Read the model definition and answer for the solid it produces. Units are mm, in the model's axes. A direction names the side the tool comes from. Give positions to 0.01 mm unless a question says otherwise; leave off trailing zeros. Loops run counter-clockwise (first coordinate to the right, second up) from the corner with the lowest first, then second, coordinate; pieces in that order, holes last. Notation, with made-up numbers: (-3, 31.25) - (37, 31.25) arc R3 cw to (37, 35.25) - close; hole circle Ø1 at (25.5, 43). An arc over 180 degrees is marked (long way). Put each result on its own line as item: value. Start each with the question number.
1. A cutting plane is placed at D-D, the plane y = -11. Determine the outline of the cut face in (x, z) (3 decimals), plus the area to 3 significant figures.
2. Given pin 1 Ø1 at (x, z) = (-6, 3) entering from -Y; pin 2 Ø3 at (y, z) = (-10.5, 7) entering from -X; pin 3 Ø1.5 at (y, z) = (4, 5.5) entering from +X; pin 4 Ø3.5 at (x, z) = (-1.5, 7) entering from +Y (3 decimals), each flat-ended and moving along its own axis, determine where each tip first touches the part or whether it passes through.
3. For faces 4 (the flat face through (-6, -3, 0)), 5 (the flat face through (5.474, 3.219, 4.829)), determine the directions among +Z, -Z, +X, -X, +Y, -Y from which every point of the face is accessible in a straight line to the end or side of a thin tool.
4. A cutting plane is placed at A-A, the plane z = 8.75. Determine the outline of the cut face in (x, y) (3 decimals), plus the area to 3 significant figures.
5. Consider L1, parallel to Y at x = -4.5, z = 0.5; L2, parallel to Y at x = 5.5, z = 5; L3, parallel to Z at x = -7, y = 13 (3 decimals). Determine where each line is inside the solid, lowest interval first. Write a range as from..to.
6. For a pull along X with two mould halves and no side action, classify faces 1 (the flat face through (-7, 11, 6.35)), 2 (the flat face through (0, 6.35, 5)), 3 (the cylindrical face through (-2.75, 12.4, 3.13)) as released by +X, released by -X, zero draft, split by the parting line, or undercut.
7. A cutting plane is placed at B-B, the plane x = 0. Determine the outline of the cut face in (y, z) (3 decimals).
8. A cutting plane is placed at C-C, the plane y = -4. Determine the outline of the cut face in (x, z) (3 decimals).
Autodesk Inventor part; units mm, degrees
ref_plane "YZ Plane" through (0, 0, 0) normal (1, 0, 0) x (0, 1, 0)
ref_plane "XZ Plane" through (0, 0, 0) normal (0, 1, 0) x (-1, 0, 0)
ref_plane "XY Plane" through (0, 0, 0) normal (0, 0, 1) x (1, 0, 0)
sketch "Sketch1" plane through (0, 0, 0) normal (0, 0, 1) x (1, 0, 0)
  circle A0 centre (0, 0) radius 12.7
  dimension "d0" = 25.4
extrude "Extrusion1" add sketch "Sketch1" along normal blind 6.35
sketch "Sketch2" plane through (0, 0, 6.35) normal (0, 0, 1) x (1, 0, 0)
  circle A0 centre (0, 0) radius 12.7
  circle A1 centre (0, 0) radius 15.875
  dimension "d3" = 31.75
extrude "Extrusion2" add sketch "Sketch2" along normal blind 3.175
sketch "Sketch3" plane through (0, 0, 6.35) normal (0, 0, 1) x (1, 0, 0)
  circle A0 centre (0, 0) radius 12.7
extrude "Extrusion3" add sketch "Sketch3" along normal blind 3.175
sketch "Sketch4" plane through (0, 0, 9.525) normal (0, 0, 1) x (1, 0, 0)
  circle A0 centre (0, 0) radius 15.875
  line L0 (3.6662, 6.35) -> (7.3323, 0)
  line L1 (7.3323, 0) -> (3.6662, -6.35)
  line L2 (3.6662, -6.35) -> (-3.6662, -6.35)
  line L3 (-3.6662, -6.35) -> (-7.3323, 0)
  line L4 (-7.3323, 0) -> (-3.6662, 6.35)
  line L5 (-3.6662, 6.35) -> (3.6662, 6.35)
  line L6 (0, 0) -> (21.004, 0)
  dimension "d8" = 12.7
extrude "Extrusion4" cut sketch "Sketch4" against normal through all contours L1 L2 L3 L4 L5 L0
properties part number "Hex bearing" material "Iron, Cast"
Return value:
1. outline: (-11.446, 6.35) - (-6.347, 6.35) - (-6.347, 0) - (6.347, 0) - (6.347, 6.35) - (11.446, 6.35) - (11.446, 9.525) - (-11.446, 9.525) - close
1. area: 153 mm2
2. pin 1: stops at y = -11.45
2. pin 2: stops at x = -13.08
2. pin 3: stops at x = 12.28
2. pin 4: stops at y = 15.875
3. face 4: -Z, +X, -X, +Y, -Y
3. face 5: +Z, -Z
4. outline: circle Ø31.75 at (0, 0); hole (-7.332, 0) - (-3.666, -6.35) - (3.666, -6.35) - (7.332, 0) - (3.666, 6.35) - (-3.666, 6.35) - close
4. area: 652 mm2
5. L1: y = -11.88..-4.91, 4.91..11.88
5. L2: y = -11.45..-3.17, 3.17..11.45
5. L3: z = 6.35..9.525
6. face 1: zero draft
6. face 2: undercut
6. face 3: split by the parting line
7. outline: (-15.875, 6.35) - (-12.7, 6.35) - (-12.7, 0) - (-6.35, 0) - (-6.35, 9.525) - (-15.875, 9.525) - close; (6.35, 0) - (12.7, 0) - (12.7, 6.35) - (15.875, 6.35) - (15.875, 9.525) - (6.35, 9.525) - close
8. outline: (-15.363, 6.35) - (-12.054, 6.35) - (-12.054, 0) - (-5.023, 0) - (-5.023, 9.525) - (-15.363, 9.525) - close; (5.023, 0) - (12.054, 0) - (12.054, 6.35) - (15.363, 6.35) - (15.363, 9.525) - (5.023, 9.525) - close
